For this review, take the finished solid that the model builds, in its own axes (mm). Face numbers are marked on the shaded views. A direction names the side the tool comes from. Give positions to 0.01 mm unless a question says otherwise; leave off trailing zeros. Order: outer loops, then holes, each group sorted by start corner. A loop starts at its lowest first (then second) coordinate and runs counter-clockwise, first axis right, second up. Notation, with made-up numbers: (75.5, -7) - (127.5, -7) arc R20 cw to (127.5, 28) - close; hole circle Ø4 at (15.25, -10.75). An arc over 180 degrees is marked (long way). One line per item, written item: value.
```python
from build123d import *

# Parameters (mm, degrees)
SKETCH_1_R           = 8
SKETCH_1_R_2         = 5.5
EXTRUDE_1_DEPTH      = 7.5
EXTRUDE_2_REACH      = 160.38
EXTRUDE_2_END_RADIUS = 8
SKETCH_2_R           = 5
SKETCH_3_W           = 30
SKETCH_3_H           = 30
EXTRUDE_3_DEPTH      = 8.61101214
SKETCH_4_R           = 1.5
CUT_EXTRUDE_1_DEPTH  = 10


with BuildPart() as part:
    # 草图1 → 凸台-拉伸1 (new, symmetric)
    with BuildSketch(Plane.XY):
        Circle(SKETCH_1_R)
        Circle(SKETCH_1_R_2, mode=Mode.SUBTRACT)
    extrude(amount=EXTRUDE_1_DEPTH, both=True)

    # 凸台-拉伸2: up to this cylinder (the profile starts outside it)
    extrude_2_end = Plane(origin=(0, 0, 0), z_dir=(0, 0, -1)) * Cylinder(EXTRUDE_2_END_RADIUS, 337.76, mode=Mode.PRIVATE)
    # 草图2 → 凸台-拉伸2 (add, up to the surface)
    with BuildSketch(Plane(origin=(0, 150, 0), x_dir=(1, 0, 0), z_dir=(0, 1, 0)), mode=Mode.PRIVATE) as extrude_2_sk1:
        with Locations(Location((0, 0, 0), (0, 0, 270))):
            Circle(SKETCH_2_R)
    extrude_2_tool1 = extrude(extrude_2_sk1.sketch, amount=-EXTRUDE_2_REACH, mode=Mode.PRIVATE) - extrude_2_end
    add(extrude_2_tool1.solids().sort_by_distance((0, 150, 0))[0])

    # 草图3 → 凸台-拉伸3 (add)
    with BuildSketch(Plane(origin=(0, 150, 0), x_dir=(1, 0, 0), z_dir=(0, 1, 0))):
        Rectangle(SKETCH_3_W, SKETCH_3_H)
    extrude(amount=EXTRUDE_3_DEPTH)

    # 草图4 → 切除-拉伸1 (cut)
    with BuildSketch(Plane(origin=(0, 158.61101214, 0), x_dir=(1, 0, 0), z_dir=(0, 1, 0))):
        with Locations(Location((12.5, -12.5, 0), (0, 0, 270))):
            Circle(SKETCH_4_R)
        with Locations(Location((12.5, 12.5, 0), (0, 0, 270))):
            Circle(SKETCH_4_R)
        with Locations(Location((-12.5, -12.5, 0), (0, 0, 270))):
            Circle(SKETCH_4_R)
        with Locations(Location((-12.5, 12.5, 0), (0, 0, 270))):
            Circle(SKETCH_4_R)
    extrude(amount=-CUT_EXTRUDE_1_DEPTH, mode=Mode.SUBTRACT)


solid = part.part
```
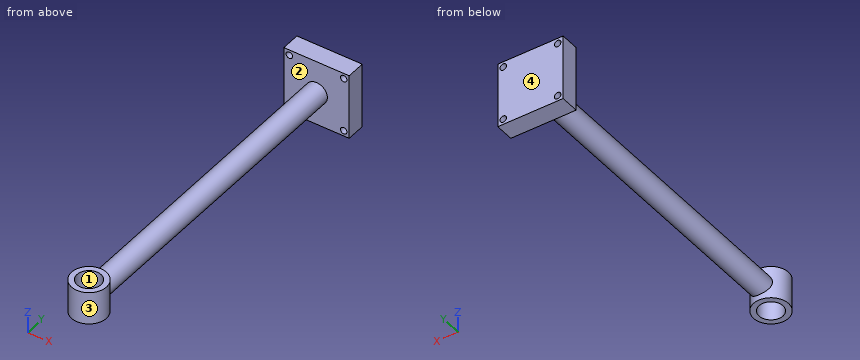
(1) Take a section at D-D (z = 0). Write out the cut boundary in (x, y) (3 decimals).
Answers below:
outline: (-15, 150) - (-5, 150) - (-5, 6.245) arc R8 ccw (long way) to (5, 6.245) - (5, 150) - (15, 150) - (15, 158.611) - (-15, 158.611) - close; hole circle Ø11 at (0, 0)
(2) Take a section at B-B (x = 12.5). Write out the cut boundary in (y, z).
Answers below:
outline: (150, -15) - (158.61, -15) - (158.61, -14) - (150, -14) - close; (150, -11) - (158.61, -11) - (158.61, 11) - (150, 11) - close; (150, 14) - (158.61, 14) - (158.61, 15) - (150, 15) - close
(3) For P1, Ø13, axis at x = -4, y = 1.5, coming from the -Z side; P2, Ø15, axis at x = 5, z = 6.5, coming from the -Y side; P3, Ø2.5, axis at x = 12.5, z = -12.5, coming from the +Y side; P4, Ø8, axis at x = -1.5, y = 3, coming from the +Z side, all flat-tipped, find the tip position at first contact; note any pin that passes through.
Answers below:
P1: stops at z = -7.5
P2: stops at y = -8
P3: passes through
P4: stops at z = 7.5
(4) Draft analysis for pull direction Y (two halves, no side actions). For the marked faces 3 and 4, state which applies: pulls with the +Y half, pulls with the -Y half, needs draft (parallel to the pull), parting line crosses it, or undercut.
Answers below:
face 3: undercut
face 4: pulls with the +Y half
(5) Wall thickness on line 1 (Y direction, x = -2.75, z = 5); line 2 (Y direction, x = -4.75, z = -6); line 3 (X direction, y = 152.75, z = 12.5): over which ranges is each line inside the solid? List them lowest first. Write a range as from..to.
Answers below:
line 1: y = -7.51..-4.76, 4.76..7.51, 150..158.61
line 2: y = -6.44..-2.77, 2.77..6.44, 150..158.61
line 3: x = -15..-14, -11..11, 14..15
(6) Take a section at C-C (y = 0). Write out the cut boundary in (x, z).
Answers below:
outline: (-8, -7.5) - (-5.5, -7.5) - (-5.5, 7.5) - (-8, 7.5) - close; (5.5, -7.5) - (8, -7.5) - (8, 7.5) - (5.5, 7.5) - close
(7) Take a section at A-A (z = 12.5). Write out the cut boundary in (x, y), then the cut area to 3 significant figures.
Answers below:
outline: (-15, 150) - (-14, 150) - (-14, 158.61) - (-15, 158.61) - close; (-11, 150) - (11, 150) - (11, 158.61) - (-11, 158.61) - close; (14, 150) - (15, 150) - (15, 158.61) - (14, 158.61) - close
area: 207 mm^2
(8) Machinability: for the marked faces 1 and 2, which of the approach directions +Z, -Z, +X, -X, +Y, -Y give a long, thin tool a straight path to every point of the face, cutting with its end or side? Answer none if there is none.
Answers below:
face 1: +Z, -Z
face 2: none
